Autodesk Inventor part; units mm, degrees
ref_plane "YZ Plane" through (0, 0, 0) normal (1, 0, 0) x (0, 1, 0)
ref_plane "XZ Plane" through (0, 0, 0) normal (0, 1, 0) x (-1, 0, 0)
ref_plane "XY Plane" through (0, 0, 0) normal (0, 0, 1) x (1, 0, 0)
sketch "Boceto1" plane through (0, 0, 0) normal (0, 0, 1) x (1, 0, 0)
  circle A0 centre (1.6193, -0.0917) radius 1.25
  circle A1 centre (5.5, -3.0198) radius 1.25
  circle A2 centre (24, -0.0198) radius 1.25
  arc A3 (23.0586, -3.0782) -> (23.1969, 3.0777) centre (24, -0.0198) ccw
  line L0 (22.2281, -2.8226) -> (23.0586, -3.0782)
  line L1 (20.0701, -5.7575) -> (22.2281, -2.8226)
  line L2 (8.358, 5.473) -> (10.9932, 5.5802) construction
  line L3 (8.2096, 5.3474) -> (8.358, 5.473)
  line L4 (21.1684, 3.7215) -> (20.8396, 4.1099)
  line L5 (20.8396, 4.1099) -> (8.358, 5.473)
  arc A4 (21.1684, 3.7215) -> (23.1969, 3.0777) centre (22.6949, 5.0137) ccw
  line L6 (6.8396, 2.5802) -> (2.3489, 2.5802)
  line L7 (20.0701, -5.7575) -> (2.3489, -5.7575)
  arc A5 (2.3489, 2.5802) -> (2.3489, -5.7575) centre (2.3489, -1.5887) ccw
  line L8 (8.358, 3.2519) -> (8.3004, 3.1922)
  line L9 (6.8605, 2.5802) -> (6.7932, 2.5802)
  arc A6 (8.358, 3.2519) -> (8.2096, 5.3474) centre (6.7321, 4.1898) ccw
  arc A7 (6.8605, 2.5802) -> (8.3004, 3.1922) centre (6.8605, 4.5802) ccw
  point P0 (21.1252, -5.0888)
  point P1 (22.1345, 2.5802)
  point P2 (7.7105, 2.5802)
  dimension "d1" = 2.5
  dimension "d33" = 2
extrude "Extrusión1" add sketch "Boceto1" along normal blind 1.2
sketch "Boceto2" plane through (0, 0, 1.2) normal (0, 0, 1) x (1, 0, 0)
  arc A0 (23.0586, -3.0782) -> (23.1969, 3.0777) centre (24, -0.0198) ccw
  line L0 (20.8396, 4.1099) -> (8.358, 5.473)
  line L1 (8.7666, 5.4284) -> (20.8396, 4.1099)
  line L2 (20.8396, 4.1099) -> (21.4572, 3.3711)
  line L3 (21.4572, 3.3711) -> (21.7914, 3.2147)
  line L4 (8.7666, 5.4284) -> (19.5399, 2.598)
  arc A1 (21.7914, 3.2147) -> (19.5399, 2.598) centre (21.6249, -0.5954) ccw
  line L5 (8.5436, -5.7575) -> (9.8539, -3.8256)
  line L6 (9.8539, -3.8256) -> (17.608, -5.2919)
  line L7 (17.3447, -5.7575) -> (8.5436, -5.7575)
  arc A2 (17.608, -5.2919) -> (17.3447, -5.7575) centre (17.7053, -5.6542) ccw
  point P0 (0, 0)
  point P1 (0.0237, -5.8)
  point P2 (24.1345, 2.6)
extrude "Extrusión2" add sketch "Boceto2" along normal blind 3.4
sketch "Boceto3" plane through (0, 0, 0) normal (0, 0, -1) x (-1, 0, 0)
  circle A0 centre (0, 0) radius 1.2362
  circle A1 centre (-5.5, -3.0198) radius 1.25
  circle A2 centre (-5.5, -3.0198) radius 1.25
  circle A3 centre (-24, -0.0198) radius 1.25
  circle A4 centre (-24, -0.0198) radius 1.25
extrude "Extrusión3" add sketch "Boceto3" against normal blind 2.5 contours A1 | A3
sketch "Boceto4" plane through (5.5, -3.0198, 2.5) normal (0, 0, 1) x (1, 0, 0)
  circle A0 centre (0, 0) radius 1.25
  circle A1 centre (0, 0) radius 1.25
  point P0 (-5.5, 3.0198)
extrude "Extrusión4" add sketch "Boceto4" along normal blind 1.5
sketch "Boceto6" plane through (0, 0, 1.2) normal (0, 0, 1) x (1, 0, 0)
  line L0 (9.8539, -3.8256) -> (17.608, -5.2919)
  line L1 (9.8539, -3.8256) -> (11.2672, 4.7714)
  line L2 (19.5399, 2.598) -> (8.7666, 5.4284)
  line L3 (11.2672, 4.7714) -> (19.5399, 2.598)
  line L4 (19.5399, 2.598) -> (15.9763, -4.9536)
  line L5 (9.8539, -3.8256) -> (8.5436, -5.7575)
  line L6 (15.9763, -4.9536) -> (9.8539, -3.8256)
  point P0 (0, 0)
extrude "Extrusión6" add sketch "Boceto6" along normal blind 3
properties part number "Pieza2_3DPrint"
Model file for the job. Use its own axes, mm. A direction names the side the tool comes from. Round coordinates to 2 decimals unless told otherwise and drop trailing zeros. Order: outer loops, then holes, each group sorted by start corner. A loop starts at its lowest first (then second) coordinate and runs counter-clockwise, first axis right, second up. Notation, with made-up numbers: M 49,81.5 L 104,81.5 A8 cw 104,90.5 Z; hole C 79,19 d3. An arc over 180 degrees is marked long. Write each question's results on one line, items separated by ' | '. Start each with the question number.
(1) Saw through at D-D, the plane x = 24. Give the cut face in (y, z).
(2) Which spindle directions (+Z, -Z, +X, -X, +Y, -Y) get a long thin tool onto all of the face, cutting with end or side? Do faces 1 (the face through (10.936, 4.858, 3.27)), 2 (the face through (5.418, -1.773, 2.269)), 3 (the face through (24, 0, 2.5)). Say none if no direction does.
(3) Saw through at C-C, the plane x = 1.5. Give the cut face in (y, z).
(4) Drop flat-ended pins along their axis: pin 1 (1.3 mm diameter, centred on x = 4.5, z = 0.5, fed in from +Y); pin 2 (1 mm diameter, centred on y = -2.5, z = 0.5, fed in from +X); pin 3 (0.8 mm diameter, centred on x = 24, y = 0, fed in from +Z); pin 4 (2 mm diameter, centred on x = 1.62, y = -0.09, fed in from +Z). Give the stop position or say it passes through.
(5) Two-plate mould, pull along Y, no slides. Class faces 4 (the face through (17.783, -1.125, 2.679)), 5 (the face through (20.6, 3.08, 2.88)), 6 (the face through (22.845, -0.499, 1.841)), 7 (the face through (12, -5, 4.6)): pulls with the +Y half, pulls with the -Y half, needs draft (parallel to the pull), parting line crosses it, or undercut.
(6) Probe probe 1 along Z at (x, y) = (18.25, -2.75); probe 2 along Z at (x, y) = (15.5, 3); probe 3 along X at (y, z) = (-2.5, 1.95). List the from-to ranges inside material, lowest first. Write a range as from..to.
(7) Saw through at B-B, the plane y = 0.5. Give the cut face in (x, z) (1 decimal), then the cut area to 3 significant figures.
Established:
1) outline: M -3.22,0 L 3.18,0 L 3.18,1.2 L 1.23,1.2 L 1.23,2.5 L -1.27,2.5 L -1.27,1.2 L -3.22,1.2 Z
2) face 1: +Z, -X | face 2: +Z | face 3: +Z, +X, +Y, -Y
3) outline: M -5.67,0 L -1.34,0 L -1.34,1.2 L -5.67,1.2 Z; M 1.15,0 L 2.49,0 L 2.49,1.2 L 1.15,1.2 Z
4) pin 1: stops at y = 2.58 | pin 2: stops at x = 26.51 | pin 3: stops at z = 2.5 | pin 4: passes through
5) face 4: undercut | face 5: pulls with the -Y half | face 6: parting line crosses it | face 7: needs draft
6) probe 1: z = 0..1.2 | probe 2: z = 0..4.2 | probe 3: x = 4.36..6.64, 10.07..17.13
7) outline: M -1.3,0 L 0.5,0 L 0.5,1.2 L -1.3,1.2 Z; M 2.7,0 L 27.2,0 L 27.2,1.2 L 25.1,1.2 L 25.1,2.5 L 22.9,2.5 L 22.9,1.2 L 18.5,1.2 L 18.5,4.2 L 10.6,4.2 L 10.6,1.2 L 2.7,1.2 Z | area: 58.4 mm^2
